Could you check a few things on this drawing? It's one solid part, dimensions in mm from its lowest x, y, z. Give positions to 0.01 mm unless a question says otherwise; leave off trailing zeros. Loops run counter-clockwise (first coordinate to the right, second up) from the corner with the lowest first, then second, coordinate; pieces in that order, holes last.
Q1. Suppose I cut it at A-A (x = 6). List the corners of the cut face in (y, z) for me (1 decimal).
Q2. I need wall thicknesses on probe 1 along Y at (x, z) = (6, 0.85) (1 decimal); probe 2 along Y at (x, z) = (11.5, 1.8) (1 decimal); probe 3 along X at (y, z) = (5.5, 0.9). Which ranges of each line are inside material? Lowest first, please.
Q3. Suppose I cut it at B-B (z = 1.3). List the corners of the cut face in (x, y) for me (1 decimal).
Q4. Thinking about a two-plate mould opening in X: for the marked faces 1, 2, 3 and 4, which applies, pulls with the +X half, pulls with the -X half, needs draft (parallel to the pull), parting line crosses it, or undercut?
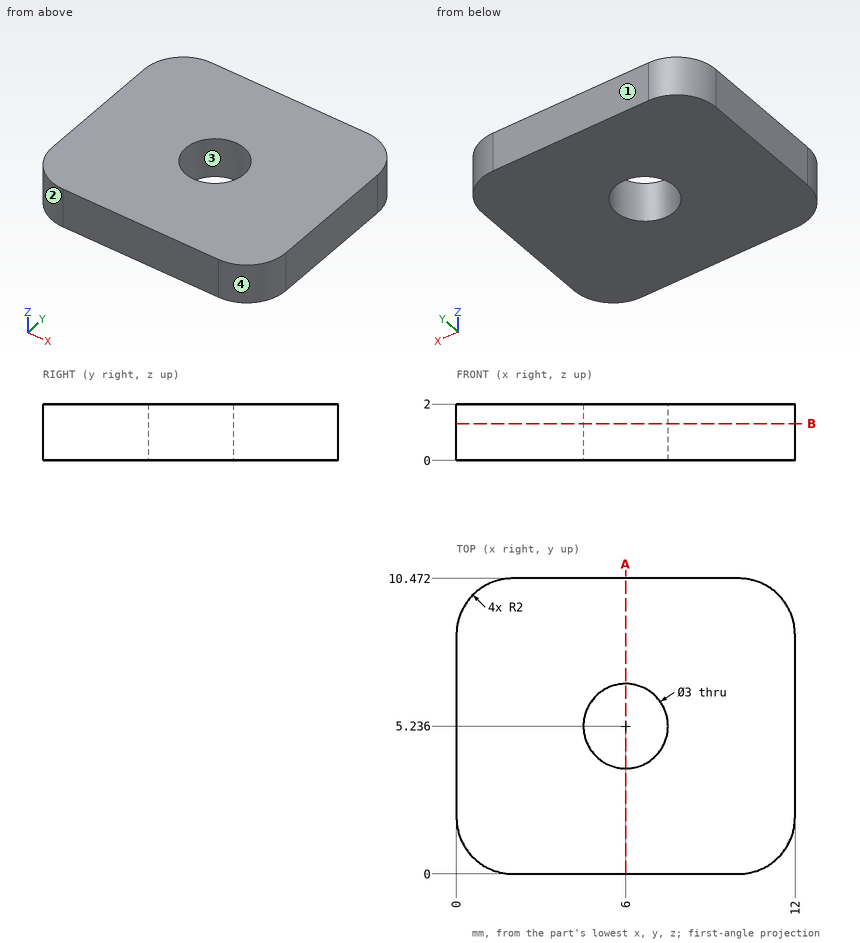
Solutions:
1. outline: (0, 0) - (3.7, 0) - (3.7, 2) - (0, 2) - close; (6.7, 0) - (10.5, 0) - (10.5, 2) - (6.7, 2) - close
2. probe 1: y = 0 to 3.7, 6.7 to 10.5
2. probe 2: y = 0.7 to 9.8
2. probe 3: x = 0 to 4.52, 7.48 to 12
3. outline: (0, 2) arc R2 ccw to (2, 0) - (10, 0) arc R2 ccw to (12, 2) - (12, 8.5) arc R2 ccw to (10, 10.5) - (2, 10.5) arc R2 ccw to (0, 8.5) - close; hole circle Ø3 at (6, 5.2)
4. face 1: needs draft
4. face 2: pulls with the -X half
4. face 3: undercut
4. face 4: pulls with the +X half
